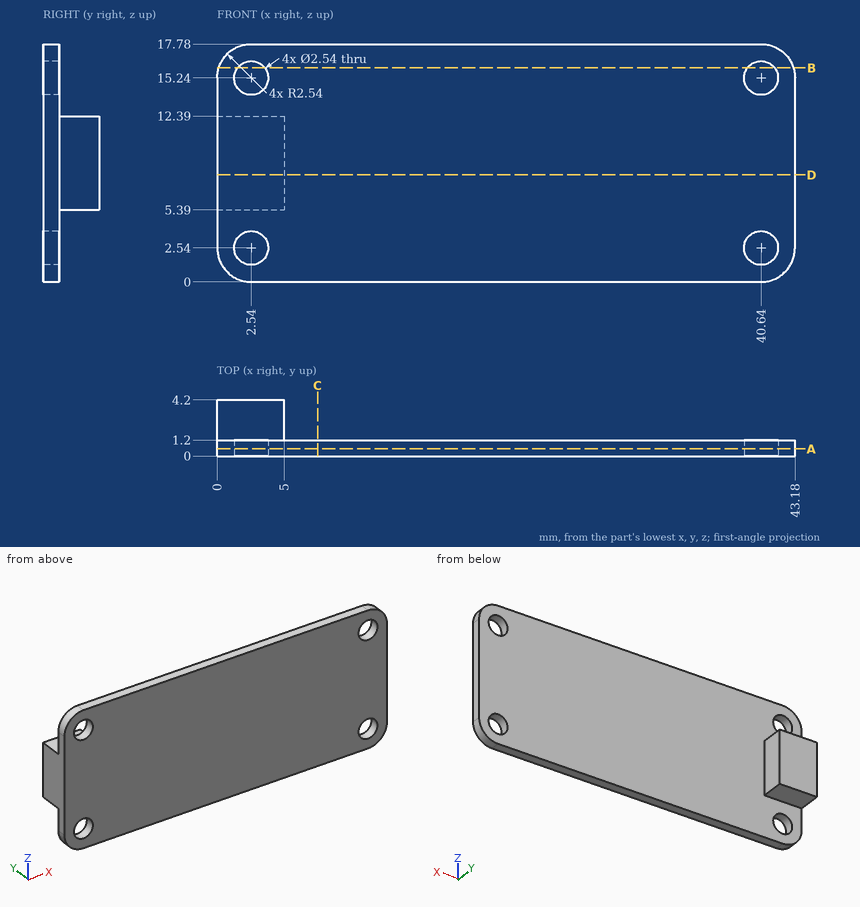
Job drawing, mm, ordinate dimensions from the low corner. One solid piece. Give positions to 0.01 mm unless a question says otherwise; leave off trailing zeros. Write each loop counter-clockwise with the first axis right and the second up, starting at its lowest first coordinate (ties: lowest second). Pieces come first, ordered by that corner, then holes. Notation, with made-up numbers: (1, 5.5) - (53, 5.5) arc R10 cw to (53, 14.5) - close; hole circle Ø5 at (-16.5, 7.25). An arc over 180 degrees is marked (long way). Answer as CSV lines item,"result".
1. Band-saw the part on D-D (z = 8). Write the cut outline in (x, y), and give its area (3 significant figures).
Responses:
outline,"(0, 0) - (43.18, 0) - (43.18, 1.2) - (5, 1.2) - (5, 4.2) - (0, 4.2) - close"
area,"66.8 mm2"
2. Band-saw the part on B-B (z = 16). Write the cut outline in (x, y).
Responses:
outline,"(0.12, 0) - (1.52, 0) - (1.52, 1.2) - (0.12, 1.2) - close; (3.56, 0) - (39.62, 0) - (39.62, 1.2) - (3.56, 1.2) - close; (41.66, 0) - (43.06, 0) - (43.06, 1.2) - (41.66, 1.2) - close"
3. Pin check, flat tips, straight feed: pin 1 (2 mm diameter, centred on x = 19, z = 3.5, fed in from +Y); pin 2 (2 mm diameter, centred on y = 3.5, z = 5.5, fed in from +X); pin 3 (2 mm diameter, centred on x = 2.54, z = 2.54, fed in from -Y); pin 4 (1.5 mm diameter, centred on x = 3, y = 3, fed in from -Z). Stop position of each tip, or through.
Responses:
pin 1,"stops at y = 1.2"
pin 2,"stops at x = 5"
pin 3,"passes through"
pin 4,"stops at z = 5.39"
4. Band-saw the part on A-A (y = 0.55). Write the cut outline in (x, z), and give its area (3 significant figures).
Responses:
outline,"(0, 2.54) arc R2.54 ccw to (2.54, 0) - (40.64, 0) arc R2.54 ccw to (43.18, 2.54) - (43.18, 15.24) arc R2.54 ccw to (40.64, 17.78) - (2.54, 17.78) arc R2.54 ccw to (0, 15.24) - close; hole circle Ø2.54 at (2.54, 2.54); hole circle Ø2.54 at (2.54, 15.24); hole circle Ø2.54 at (40.64, 2.54); hole circle Ø2.54 at (40.64, 15.24)"
area,"742 mm2"
5. Drill centre lines: L1, parallel to X at y = 0.55, z = 2.54; L2, parallel to X at y = 0.55, z = 3.5; L3, parallel to X at y = 3.2, z = 7. Where is each one in solid material? Low to high. Write a range as [from, to].
Responses:
L1,"x = [0, 1.27], [3.81, 39.37], [41.91, 43.18]"
L2,"x = [0, 1.71], [3.37, 39.81], [41.47, 43.18]"
L3,"x = [0, 5]"
6. Band-saw the part on C-C (x = 7.5). Write the cut outline in (y, z), and give its area (3 significant figures).
Responses:
outline,"(0, 0) - (1.2, 0) - (1.2, 17.78) - (0, 17.78) - close"
area,"21.3 mm2"
